```python
from build123d import *

# Parameters (mm, degrees)
SKETCH1_W            = 35
SKETCH1_H            = 105
BOSS_EXTRUDE1_DEPTH  = 6
M4_CLEARANCE_HOLE1_D = 4.8
LPATTERN2_COUNT      = 2
LPATTERN2_PITCH      = 10
SKETCH5_W            = 4.8
SKETCH5_H            = 10
SKETCH5_W_2          = 4.730666207
SKETCH5_H_2          = 10.572708501
CUT_EXTRUDE1_DEPTH   = 88.085432636
SKETCH6_W            = 11.2
SKETCH6_H            = 11.2
CUT_EXTRUDE2_DEPTH   = 4
SKETCH7_W            = 7
SKETCH7_H            = 7
CUT_EXTRUDE3_DEPTH   = 87.970527062
SKETCH8_W            = 6
SKETCH8_H            = 16.2
CUT_EXTRUDE4_DEPTH   = 4
FILLET1_R            = 10
CUT_EXTRUDE5_START   = -6
SKETCH9_W            = 37.049954943
SKETCH9_H            = 41
CUT_EXTRUDE5_DEPTH   = 3
FILLET2_R            = 30
FILLET3_R            = 30
FILLET4_R            = 1


with BuildPart() as part:
    # Sketch1 → Boss-Extrude1 (new body)
    with BuildSketch(Plane(origin=(0, 0, 0), x_dir=(1, 0, 0), z_dir=(0, 1, 0))):
        with Locations((0.111940299, -32.574626866)):
            Rectangle(SKETCH1_W, SKETCH1_H)
    extrude(amount=BOSS_EXTRUDE1_DEPTH)

    # M4 Clearance Hole1 (through all)
    with Locations(Plane(origin=(0, 6, 0), x_dir=(1, 0, 0), z_dir=(0, 1, 0))):
        with Locations((-12.388059701, 14.925373134), (12.611940299, 14.925373134), (12.611940299, -10.074626866), (-12.388059701, -10.074626866)):
            m4_clearance_hole1 = Hole(M4_CLEARANCE_HOLE1_D / 2)

    # LPattern2: M4 Clearance Hole1 ×2
    with Locations(*[(0, 0, i * LPATTERN2_PITCH) for i in range(1, LPATTERN2_COUNT)]):
        add(m4_clearance_hole1, mode=Mode.SUBTRACT)

    # Sketch5 → Cut-Extrude1 (cut, through all)
    with BuildSketch(Plane(origin=(0, 6, 0), x_dir=(1, 0, 0), z_dir=(0, 1, 0))):
        with Locations((-12.388059701, 9.925373134)):
            Rectangle(SKETCH5_W, SKETCH5_H)
        with Locations((-12.388059701, -15.074626866)):
            Rectangle(SKETCH5_W, SKETCH5_H)
        with Locations((12.577273403, 9.639018884)):
            Rectangle(SKETCH5_W_2, SKETCH5_H_2)
        with Locations((12.577273403, -15.360981116)):
            Rectangle(SKETCH5_W_2, SKETCH5_H_2)
    extrude(amount=-CUT_EXTRUDE1_DEPTH, mode=Mode.SUBTRACT)

    # Sketch6 → Cut-Extrude2 (cut)
    with BuildSketch(Plane(origin=(0, 6, 0), x_dir=(1, 0, 0), z_dir=(0, 1, 0))):
        with Locations((0.111940299, -75.074626866)):
            Rectangle(SKETCH6_W, SKETCH6_H)
    extrude(amount=-CUT_EXTRUDE2_DEPTH, mode=Mode.SUBTRACT)

    # Sketch7 → Cut-Extrude3 (cut, through all)
    with BuildSketch(Plane(origin=(0, 2, 0), x_dir=(1, 0, 0), z_dir=(0, 1, 0))):
        with Locations((0.111940299, -75.074626866)):
            Rectangle(SKETCH7_W, SKETCH7_H)
    extrude(amount=-CUT_EXTRUDE3_DEPTH, mode=Mode.SUBTRACT)

    # Sketch8 → Cut-Extrude4 (cut)
    with BuildSketch(Plane(origin=(0, 6, 0), x_dir=(1, 0, 0), z_dir=(0, 1, 0))):
        with Locations((0.111940299, -75.074626866)):
            Rectangle(SKETCH8_W, SKETCH8_H)
    extrude(amount=-CUT_EXTRUDE4_DEPTH, mode=Mode.SUBTRACT)

    # Fillet1
    fillet1_edges = [part.edges().sort_by_distance(p)[0] for p in [
        (17.611940299, 3, 85.074626866),
        (-17.388059701, 3, 85.074626866),
    ]]
    fillet(fillet1_edges, radius=FILLET1_R)

    # Sketch9 → Cut-Extrude5 (cut)
    with BuildSketch(Plane.XZ.offset(CUT_EXTRUDE5_START)):
        with Locations((1.136917771, 64.574626866)):
            Rectangle(SKETCH9_W, SKETCH9_H)
    extrude(amount=CUT_EXTRUDE5_DEPTH, mode=Mode.SUBTRACT)

    # Fillet2
    # the kernel refuses this fillet: 30 mm, written as the material it adds along each edge
    with BuildSketch(Plane(origin=(-17.388059701, 3, 44.074626866), x_dir=(0, 1, 0), z_dir=(1, 0, 0))) as fillet2_piece_1:
        with BuildLine():
            CenterArc((30, 13.076696831), FILLET2_R, 180, 25.841932763)
            Line((0, 13.076696831), (-0.6, 13.076696831))
            Line((-0.6, 13.076696831), (-0.6, 0))
            Line((-0.6, 0), (0, -0.6))
            ThreePointArc((0, -0.6), (1.5, -0.6), (2.46, -0.261533937))
            Line((2.46, -0.261533937), (3, 0))
        make_face()
    extrude(amount=35)

    # Fillet3
    fillet3_edges = [part.edges().sort_by_distance(p)[0] for p in [
        (0.111940299, 6, 44.074626866),
    ]]
    fillet(fillet3_edges, radius=FILLET3_R)

    # Fillet4
    fillet4_edges = [part.edges().sort_by_distance(p)[0] for p in [
        (-17.388059701, 3, -19.925373134),
        (17.611940299, 3, -19.925373134),
    ]]
    fillet(fillet4_edges, radius=FILLET4_R)


solid = part.part
```
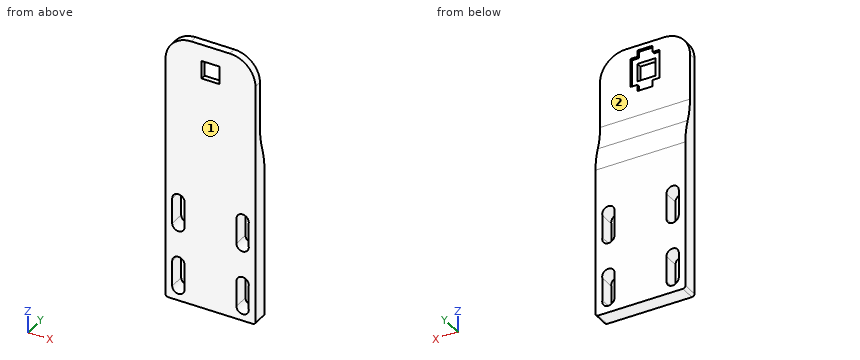
Build history of the part. All positions in model axes, mm. Face numbers are marked on the shaded views. A direction names the side the tool comes from. Coordinates: 2 decimals unless noted, no trailing zeros. Order: outer loops, then holes, each group sorted by start corner. A loop starts at its lowest first (then second) coordinate and runs counter-clockwise, first axis right, second up. Notation, with made-up numbers: (33, 20.25) -> (86, 20.25) arc R36 ccw to (86, 54.25) -> close; hole circle Ø9 at (70.5, -10). An arc over 180 degrees is marked (long way). Answer in a Markdown table with one row per item. Add a question column.
Q1. Band-saw the part on C-C, the plane z = 50. List the corners of the cut face in (x, y).
Q2. Band-saw the part on D-D, the plane x = 9. List the corners of the cut face in (y, z).
Q3. Wall check: line 1 along X through (y, z) = (1.15, -7); line 2 along Z through (x, y) = (5, 2.9); line 3 along Z through (x, y) = (-0.5, 0.5). Give the ranges that are in metal, low to high. Write a range as [from, to].
Q4. Band-saw the part on B-B, the plane x = 4.5. List the corners of the cut face in (y, z).
Q5. Which spindle directions (+Z, -Z, +X, -X, +Y, -Y) get a long thin tool onto all of the face, cutting with end or side? Do the marked faces 1 and 2. Say none if no direction does.
Q6. Drop flat-ended pins along their axis: pin 1 (0.5 mm diameter, centred on y = 2.5, z = 76, fed in from -X); pin 2 (6 mm diameter, centred on x = 12.61, z = 10.07, fed in from -Y); pin 3 (8.5 mm diameter, centred on x = 3, z = 64.5, fed in from +Y); pin 4 (1.1 mm diameter, centred on y = 2.5, z = 76, fed in from +X). Give the stop position or say it passes through.
Q7. Band-saw the part on A-A, the plane z = 13. List the corners of the cut face in (x, y), then the cut area to 3 significant figures.
Answers follow:
| question | item | result |
|---|---|---|
| 1 | outline | (-17.39, 0) -> (17.61, 0) -> (17.61, 3.86) -> (-17.39, 3.86) -> close |
| 2 | outline | (0, -19.93) -> (6, -19.93) -> (6, 38.42) arc R30 ccw to (4.5, 47.78) arc R30 cw to (3, 57.15) -> (3, 84.98) -> (0, 84.98) -> close |
| 3 | line 1 | [-17.39, -14.79], [-9.99, 10.21], [14.94, 17.61] |
| 3 | line 2 | [-19.93, 69.47], [80.67, 85.07] |
| 3 | line 3 | [-19.93, 71.57], [78.57, 85.07] |
| 4 | outline | (0, -19.93) -> (6, -19.93) -> (6, 38.42) arc R30 ccw to (4.5, 47.78) arc R30 cw to (3, 57.15) -> (3, 69.47) -> (2, 69.47) -> (2, 80.67) -> (3, 80.67) -> (3, 85.07) -> (0, 85.07) -> close |
| 5 | face 1 | +Z, -Z, +X, -X, -Y |
| 5 | face 2 | +Z, +X, -X, +Y |
| 6 | pin 1 | x = -17.37 |
| 6 | pin 2 | y = 0 |
| 6 | pin 3 | y = 3 |
| 6 | pin 4 | x = 17.6 |
| 7 | outline | (-17.39, 0) -> (-14.79, 0) -> (-14.79, 6) -> (-17.39, 6) -> close; (-9.99, 0) -> (10.21, 0) -> (10.21, 6) -> (-9.99, 6) -> close; (14.94, 0) -> (17.61, 0) -> (17.61, 6) -> (14.94, 6) -> close |
| 7 | area | 153 mm^2 |
